Autodesk Inventor part; units mm, degrees
ref_plane "YZ Plane" through (0, 0, 0) normal (1, 0, 0) x (0, 1, 0)
ref_plane "XZ Plane" through (0, 0, 0) normal (0, 1, 0) x (-1, 0, 0)
ref_plane "XY Plane" through (0, 0, 0) normal (0, 0, 1) x (1, 0, 0)
sketch "Sketch1" plane through (0, 0, 0) normal (0, 0, 1) x (1, 0, 0)
  line L0 (0, 0) -> (-20, 0)
  line L1 (-20, 0) -> (-20, 10)
  line L2 (-20, 10) -> (-26, 10)
  line L3 (-26, 10) -> (-26, 18)
  line L4 (-26, 18) -> (-20, 18)
  line L5 (-20, 18) -> (-20, 28)
  line L6 (-20, 28) -> (-26, 28)
  line L7 (-26, 28) -> (-26, 36)
  line L8 (-26, 36) -> (-20, 36)
  line L9 (-20, 36) -> (-20, 46)
  line L10 (-20, 46) -> (-26, 46)
  line L11 (-26, 46) -> (-26, 54)
  line L12 (-26, 54) -> (-20, 54)
  line L13 (-20, 54) -> (-20, 64)
  line L14 (-20, 64) -> (-26, 64)
  line L15 (-26, 64) -> (-26, 72)
  line L16 (-26, 72) -> (-20, 72)
  line L17 (-20, 72) -> (-20, 82)
  line L18 (-20, 82) -> (-26, 82)
  line L19 (-26, 82) -> (-26, 90)
  line L20 (-26, 90) -> (-20, 90)
  line L21 (-20, 90) -> (-20, 117)
  line L22 (-20, 117) -> (0, 117)
  line L23 (0, 117) -> (0, 0) construction
  line L24 (0, 0) -> (20, 0)
  line L25 (20, 0) -> (20, 10)
  line L26 (20, 10) -> (26, 10)
  line L27 (26, 10) -> (26, 18)
  line L28 (26, 18) -> (20, 18)
  line L29 (20, 18) -> (20, 28)
  line L30 (26, 28) -> (26, 36)
  line L31 (26, 36) -> (20, 36)
  line L32 (20, 36) -> (20, 46)
  line L33 (20, 46) -> (26, 46)
  line L34 (26, 46) -> (26, 54)
  line L35 (26, 54) -> (20, 54)
  line L36 (20, 54) -> (20, 64)
  line L37 (20, 64) -> (26, 64)
  line L38 (26, 64) -> (26, 72)
  line L39 (26, 72) -> (20, 72)
  line L40 (20, 72) -> (20, 82)
  line L41 (20, 82) -> (26, 82)
  line L42 (26, 82) -> (26, 90)
  line L43 (26, 90) -> (20, 90)
  line L44 (20, 90) -> (20, 117)
  line L45 (20, 117) -> (0, 117)
  line L46 (20, 28) -> (26, 28)
  point P0 (-23, 90)
  dimension "d18" = 20
  dimension "d20" = 6
  dimension "d21" = 8
  dimension "d22" = 10
  dimension "d23" = 6
  dimension "d24" = 8
  dimension "d25" = 117
  dimension "d33" = 8
  dimension "d34" = 8
  dimension "d35" = 8
  dimension "d36" = 10
  dimension "d37" = 10
  dimension "d38" = 10
  dimension "d39" = 20
  dimension "d42" = 90
extrude "Extrusion1" add sketch "Sketch1" along normal blind 6
properties part number "sort support wall 2"
Part model, mm, in its own coordinate system. A direction names the side the tool comes from. Coordinates: 2 decimals unless noted, no trailing zeros. Return JSON: item names as keys, results as strings. Group by question number.
Item 1: Pull direction Y, two halves, no side cores. Call faces 5 (the face through (-23, 18, 3)), 6 (the face through (23, 18, 3)), 7 (the face through (20, 5, 3)), 8 (the face through (23, 10, 3)): pulls with the +Y half, pulls with the -Y half, needs draft (parallel to the pull), parting line crosses it, or undercut.
Item 2: Which spindle directions (+Z, -Z, +X, -X, +Y, -Y) get a long thin tool onto all of the face, cutting with end or side? Do faces 1 (the face through (-23, 64, 3)), 2 (the face through (20, 77, 3)), 3 (the face through (23, 90, 3)), 4 (the face through (-23, 90, 3)). Say none if no direction does.
Item 3: Drill centre lines: probe 1 along Y at (x, z) = (-21, 0.3); probe 2 along X at (y, z) = (37, 4.15). Where is each one in solid material? Low to high. Write a range as from..to.
Item 4: Pin check, flat tips, straight feed: pin 1 (3 mm diameter, centred on x = -22, z = 4.5, fed in from -Y); pin 2 (1.5 mm diameter, centred on y = 100, z = 4.5, fed in from +X); pin 3 (3 mm diameter, centred on y = 24.5, z = 3, fed in from -X). Stop position of each tip, or through.
Check values:
{
 "1": {"face 5": "undercut", "face 6": "undercut", "face 7": "needs draft", "face 8": "pulls with the -Y half"},
 "2": {"face 1": "+Z, -Z, -X", "face 2": "+Z, -Z, +X", "face 3": "+Z, -Z, +X, +Y", "face 4": "+Z, -Z, -X, +Y"},
 "3": {"probe 1": "y = 10..18, 28..36, 46..54, 64..72, 82..90", "probe 2": "x = -20..20"},
 "4": {"pin 1": "stops at y = 10", "pin 2": "stops at x = 20", "pin 3": "stops at x = -20"}
}
